Geometry: final body of the model. Coordinates: model frame, mm. Give positions to 0.01 mm unless a question says otherwise; leave off trailing zeros. Write each loop counter-clockwise with the first axis right and the second up, starting at its lowest first coordinate (ties: lowest second). Pieces come first, ordered by that corner, then holes. Notation, with made-up numbers: M 3.25,-40 L 59.25,-40 A7 ccw 59.25,-35 Z; hole C -36,55 d9. An arc over 180 degrees is marked long. One line per question, with ' | ' between items.
Autodesk Inventor part; units mm, degrees
ref_plane "YZ Plane" through (0, 0, 0) normal (1, 0, 0) x (0, 1, 0)
ref_plane "XZ Plane" through (0, 0, 0) normal (0, 1, 0) x (-1, 0, 0)
ref_plane "XY Plane" through (0, 0, 0) normal (0, 0, 1) x (1, 0, 0)
sketch "Sketch1" plane through (0, 0, 0) normal (0, 0, 1) x (1, 0, 0)
  line L0 (69.85, -19.05) -> (-69.85, -19.05)
  line L1 (-69.85, -19.05) -> (-69.85, 19.05)
  line L2 (-69.85, 19.05) -> (69.85, 19.05)
  line L3 (69.85, 19.05) -> (69.85, -19.05)
  line L4 (69.85, -19.05) -> (-69.85, 19.05) construction
  line L5 (-69.85, -19.05) -> (69.85, 19.05) construction
  point P0 (0, 0)
  dimension "d0" = 139.7
  dimension "d1" = 38.1
extrude "Extrusion1" add sketch "Sketch1" along normal blind 6.35
sketch "Sketch2" plane through (0, 0, 6.35) normal (0, 0, 1) x (1, 0, 0)
  line L0 (-69.85, 19.05) -> (-69.85, -19.05)
  line L1 (69.85, 19.05) -> (-69.85, 19.05)
  point P0 (0, 0)
  point P1 (-57.15, 6.35)
  point P2 (-44.45, 6.35)
  point P3 (-31.75, 6.35)
  point P4 (-69.85, 0)
  dimension "d5" = 12.7
  dimension "d6" = 12.7
  dimension "d14" = 12.7
  dimension "d15" = 12.7
hole "Hole1" at (-57.15, 6.35, 6.35) at (-44.45, 6.35, 6.35) at (-31.75, 6.35, 6.35) direction (0, 0, -1) diameter 3.9624 end through all
sketch "Sketch3" plane through (0, 0, 6.35) normal (0, 0, 1) x (1, 0, 0)
  line L0 (69.85, 19.05) -> (-69.85, 19.05)
  line L1 (-69.85, -19.05) -> (69.85, -19.05)
  line L2 (69.85, -19.05) -> (69.85, 19.05)
  line L3 (6.35, -9.525) -> (57.15, -9.525) construction
  line L4 (-69.85, 19.05) -> (-69.85, -19.05) construction
  point P0 (0, 0)
  point P1 (66.675, 12.7)
  point P2 (66.675, -12.7)
  point P3 (-69.85, 0)
  dimension "d16" = 6.35
  dimension "d17" = 6.35
  dimension "d18" = 3.175
  dimension "d39" = 50.8
  dimension "d41" = 28.575
  dimension "d43" = 12.7
hole "Hole2" at (66.675, 12.7, 6.35) at (66.675, -12.7, 6.35) at (6.35, -9.525, 6.35) at (57.15, -9.525, 6.35) direction (0, 0, -1) diameter 4.318 end through all
sketch "Sketch6" plane through (0, 0, 6.35) normal (0, 0, 1) x (1, 0, 0)
  line L0 (47.75, 9.525) -> (15.75, 9.525) construction
  line L1 (69.85, -19.05) -> (69.85, 19.05) construction
  line L2 (-69.85, -19.05) -> (69.85, -19.05) construction
  point P0 (0, 0)
  point P1 (69.85, 0)
  point P2 (69.85, 0)
  point P3 (31.75, 9.525)
  point P4 (31.75, 1.524)
  dimension "d30" = 32
  dimension "d45" = 28.575
  dimension "d46" = 38.1
  dimension "d47" = 8.001
hole "Hole3" at (47.75, 9.525, 6.35) at (15.75, 9.525, 6.35) at (31.75, 9.525, 6.35) direction (0, 0, -1) diameter 2.459 end through all
properties part number "EL2-021" material "Aluminum 6061"
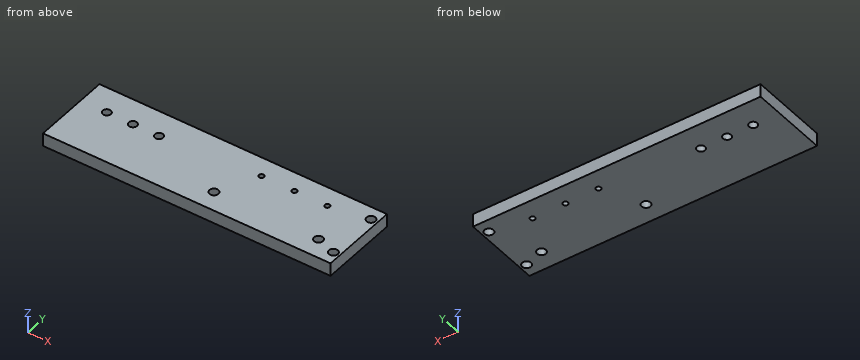
(1) Cut plane D-D, the plane z = 1. Count the separate pieces of the cut face and the enclosed holes in it, then the cut area to 3 significant figures.
Working result:
separate pieces: 1 | enclosed holes: 10 | area: 5,210 mm^2
(2) Cut plane A-A, the plane y = 12.7. Return loops of the section in (x, z).
Working result:
outline: M -69.85,0 L 64.52,0 L 64.52,6.35 L -69.85,6.35 Z; M 68.83,0 L 69.85,0 L 69.85,6.35 L 68.83,6.35 Z
(3) Cut plane C-C, the plane y = 6.35. Return loops of the section in (x, z), then the cut area to 3 significant figures.
Working result:
outline: M -69.85,0 L -59.13,0 L -59.13,6.35 L -69.85,6.35 Z; M -55.17,0 L -46.43,0 L -46.43,6.35 L -55.17,6.35 Z; M -42.47,0 L -33.73,0 L -33.73,6.35 L -42.47,6.35 Z; M -29.77,0 L 69.85,0 L 69.85,6.35 L -29.77,6.35 Z | area: 812 mm^2
(4) Material intervals for L1, parallel to X at y = 6.35, z = 2; L2, parallel to Y at x = -31.75, z = 4.5; L3, parallel to X at y = -12.7, z = 2.25, sorted ascending. Write a range as [from, to].
Working result:
L1: x = [-69.85, -59.13], [-55.17, -46.43], [-42.47, -33.73], [-29.77, 69.85] | L2: y = [-19.05, 4.37], [8.33, 19.05] | L3: x = [-69.85, 64.52], [68.83, 69.85]
(5) First-contact query: P1, Ø3.5, axis at x = 6.35, y = -9.525, coming from the -Z side. Flat tip, straight axial feed; report the tip coordinate or a pass-through.
Working result:
P1: passes through
(6) Cut plane B-B, the plane x = 47.75. Return loops of the section in (y, z), then the cut area to 3 significant figures.
Working result:
outline: M -19.05,0 L 8.3,0 L 8.3,6.35 L -19.05,6.35 Z; M 10.75,0 L 19.05,0 L 19.05,6.35 L 10.75,6.35 Z | area: 226 mm^2
